```python
from build123d import *

# Parameters (mm, degrees)
SKETCH1_R                    = 4
SKETCH1_R_2                  = 1.5
EXTRUDE1_DEPTH               = 2
SKETCHED_START               = -63
SKETCHED_BEND1_OUTLINE_W     = 20
SKETCHED_BEND1_OUTLINE_H     = 2
SKETCHED_BEND1_DEPTH         = 35
SKETCHED_START_2             = -27.76405
SKETCHED_BEND1_2_OUTLINE_R   = 1.5
SKETCHED_BEND1_2_OUTLINE_R_2 = 4
SKETCHED_BEND1_2_DEPTH       = 1.76405
SKETCHED_START_3             = -28
SKETCHED_BEND1_3_OUTLINE_R   = 1.5
SKETCHED_BEND1_3_OUTLINE_R_2 = 4
SKETCHED_BEND1_3_DEPTH       = 2.5
SKETCHED_START_4             = -11
SKETCHED_BEND1_4_DEPTH       = 22


with BuildPart() as part:
    # Sketch1 → Extrude1 (new body)
    with BuildSketch(Plane.XY):
        with BuildLine():
            Line((0, -3), (0, -10))
            Line((0, -10), (-52, -10))
            ThreePointArc((-52, -10), (-62, 0), (-52, 10))
            Line((-52, 10), (0, 10))
            Line((0, 10), (0, 3))
            ThreePointArc((0, 3), (-3, 0), (0, -3))
        make_face()
        with Locations((-52, 0)):
            Circle(SKETCH1_R, mode=Mode.SUBTRACT)
        with Locations((-45, 0)):
            Circle(SKETCH1_R_2, mode=Mode.SUBTRACT)
        with Locations((-47.050252532, -4.949747468)):
            Circle(SKETCH1_R_2, mode=Mode.SUBTRACT)
        with Locations((-52, -7)):
            Circle(SKETCH1_R_2, mode=Mode.SUBTRACT)
        with Locations((-59, 0)):
            Circle(SKETCH1_R_2, mode=Mode.SUBTRACT)
        with Locations((-52, 7)):
            Circle(SKETCH1_R_2, mode=Mode.SUBTRACT)
        with Locations((-47.050252532, 4.949747468)):
            Circle(SKETCH1_R_2, mode=Mode.SUBTRACT)
        with Locations((-4.95, -4.95)):
            Circle(SKETCH1_R_2, mode=Mode.SUBTRACT)
        with Locations((-14.85, -4.95)):
            Circle(SKETCH1_R_2, mode=Mode.SUBTRACT)
        with Locations(Location((-4.95, 4.95, 0), (0, 0, 180))):
            Circle(SKETCH1_R_2, mode=Mode.SUBTRACT)
        with Locations(Location((-14.85, 4.95, 0), (0, 0, 180))):
            Circle(SKETCH1_R_2, mode=Mode.SUBTRACT)
    extrude(amount=EXTRUDE1_DEPTH)

    # Sketched Bend1: read off the stored shape, not the designer's step
    # Sketched Bend1 outline → Sketched Bend1 (cut)
    with BuildSketch(Plane.YZ.offset(SKETCHED_START)):
        with Locations((0, 1)):
            Rectangle(SKETCHED_BEND1_OUTLINE_W, SKETCHED_BEND1_OUTLINE_H)
    extrude(amount=SKETCHED_BEND1_DEPTH, mode=Mode.SUBTRACT)

    # Sketched Bend1 2 outline → Sketched Bend1 2 (add)
    with BuildSketch(Plane.YZ.offset(SKETCHED_START_2)):
        with BuildLine():
            Line((10, 2), (10, 26.64380551))
            ThreePointArc((10, 26.64380551), (0, 36.64380551), (-10, 26.64380551))
            Line((-10, 26.64380551), (-10, 2))
            Line((-10, 2), (10, 2))
        make_face()
        with Locations((-7, 26.64380551)):
            Circle(SKETCHED_BEND1_2_OUTLINE_R, mode=Mode.SUBTRACT)
        with Locations((-4.949747468, 21.694058042)):
            Circle(SKETCHED_BEND1_2_OUTLINE_R, mode=Mode.SUBTRACT)
        with Locations((0, 19.64380551)):
            Circle(SKETCHED_BEND1_2_OUTLINE_R, mode=Mode.SUBTRACT)
        with Locations((4.949747468, 21.694058042)):
            Circle(SKETCHED_BEND1_2_OUTLINE_R, mode=Mode.SUBTRACT)
        with Locations((0, 26.64380551)):
            Circle(SKETCHED_BEND1_2_OUTLINE_R_2, mode=Mode.SUBTRACT)
        with Locations((7, 26.64380551)):
            Circle(SKETCHED_BEND1_2_OUTLINE_R, mode=Mode.SUBTRACT)
        with Locations((0, 33.64380551)):
            Circle(SKETCHED_BEND1_2_OUTLINE_R, mode=Mode.SUBTRACT)
    extrude(amount=SKETCHED_BEND1_2_DEPTH)

    # Sketched Bend1 3 outline → Sketched Bend1 3 (add)
    with BuildSketch(Plane.YZ.offset(SKETCHED_START_3)):
        with BuildLine():
            Line((10, 2), (10, 26.64380551))
            ThreePointArc((10, 26.64380551), (0, 36.64380551), (-10, 26.64380551))
            Line((-10, 26.64380551), (-10, 2))
            Line((-10, 2), (10, 2))
        make_face()
        with Locations((-7, 26.64380551)):
            Circle(SKETCHED_BEND1_3_OUTLINE_R, mode=Mode.SUBTRACT)
        with Locations((-4.949747468, 21.694058042)):
            Circle(SKETCHED_BEND1_3_OUTLINE_R, mode=Mode.SUBTRACT)
        with Locations((0, 19.64380551)):
            Circle(SKETCHED_BEND1_3_OUTLINE_R, mode=Mode.SUBTRACT)
        with Locations((4.949747468, 21.694058042)):
            Circle(SKETCHED_BEND1_3_OUTLINE_R, mode=Mode.SUBTRACT)
        with Locations((0, 26.64380551)):
            Circle(SKETCHED_BEND1_3_OUTLINE_R_2, mode=Mode.SUBTRACT)
        with Locations((7, 26.64380551)):
            Circle(SKETCHED_BEND1_3_OUTLINE_R, mode=Mode.SUBTRACT)
        with Locations((0, 33.64380551)):
            Circle(SKETCHED_BEND1_3_OUTLINE_R, mode=Mode.SUBTRACT)
    extrude(amount=SKETCHED_BEND1_3_DEPTH)

    # Sketched Bend1 4 outline → Sketched Bend1 4 (cut)
    with BuildSketch(Plane(origin=(0, 0, 0), x_dir=(1, 0, 0), z_dir=(0, 1, 0)).offset(SKETCHED_START_4)):
        with BuildLine():
            Line((-26, -2.5), (-26, -38))
            Line((-26, -38), (-25.5, -38))
            Line((-25.5, -38), (-25.5, -2))
            ThreePointArc((-25.5, -2), (-25.853553391, -2.146446609), (-26, -2.5))
        make_face()
        with BuildLine():
            Line((-29, -38), (-27.999999998, -38))
            Line((-27.999999998, -38), (-28, -2.5))
            ThreePointArc((-28, -2.5), (-27.267766953, -0.732233047), (-25.5, 0))
            Line((-25.5, 0), (-24, 0))
            Line((-24, 0), (-24, 1))
            Line((-24, 1), (-29, 1))
            Line((-29, 1), (-29, -38))
        make_face()
    extrude(amount=SKETCHED_BEND1_4_DEPTH, mode=Mode.SUBTRACT)

    # Mirror1: part across plane


with BuildPart() as part_1:
    add(part.part)
    add(part.part.mirror(Plane(origin=(0, -3, 2), x_dir=(0, 0, 1), z_dir=(-1, 0, 0))))


solid = part_1.part
```
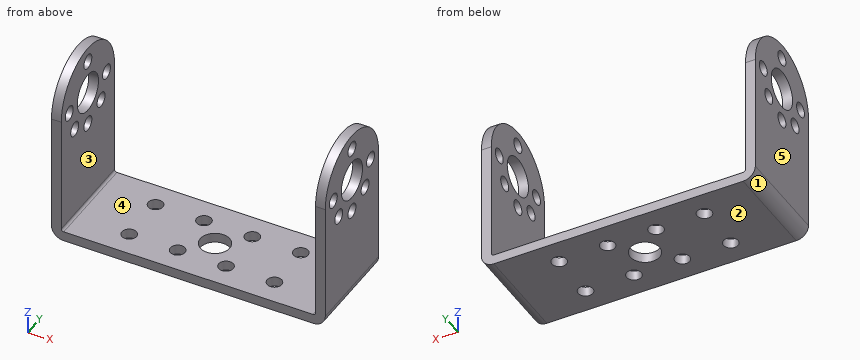
Work out the finished part from the listing and answer in its coordinate system (mm). Face numbers are marked on the shaded views. A direction names the side the tool comes from. Give positions to 0.01 mm unless a question says otherwise; leave off trailing zeros. Order: outer loops, then holes, each group sorted by start corner. A loop starts at its lowest first (then second) coordinate and runs counter-clockwise, first axis right, second up. Notation, with made-up numbers: (51, 59) - (107, 59) arc R25 ccw to (107, 82) - close; hole circle Ø8 at (53, 17). An arc over 180 degrees is marked (long way). One line per item, written item: value. Start each with the question number.
1. Section D-D, the plane y = 0 is taken. Count the separate pieces of the cut face and the enclosed holes in it, then the cut area to 3 significant figures.
2. Section C-C, the plane y = 7.75 is taken. Write down the section's boundary in (x, z), then the cut area to 3 significant figures.
3. Section B-B, the plane z = 11 is taken. Write down the section's boundary in (x, y), then the cut area to 3 significant figures.
4. Section A-A, the plane x = 14.85 is taken. Write down the section's boundary in (y, z), then the cut area to 3 significant figures.
5. This flat-tipped pin is pushed along its axis until it touches: pin 1 Ø6 at (x, y) = (5, -4) entering from +Z. Where does it stop, or does it pass through?
6. Consider line 1 (Y direction, x = -4.95, z = 1.65); line 2 (X direction, y = -1, z = 3.5); line 3 (X direction, y = 4.95, z = 0.7). Determine where each line is inside the solid, lowest interval first.
7. For a pull along X with two mould halves and no side action, classify the marked faces 1, 2 and 3 as released by +X, released by -X, zero draft, split by the parting line, or undercut.
8. Which of the six approach directions +Z, -Z, +X, -X, +Y, -Y give full straight-line access (tool end or side, diameter ignored) to the marked faces 4 and 5?
Filled sheet:
1. separate pieces: 8
1. enclosed holes: 0
1. area: 180 mm²
2. outline: (-28, 2.5) arc R2.5 ccw to (-25.5, 0) - (25.5, 0) arc R2.5 ccw to (28, 2.5) - (28, 25.34) - (26, 25.34) - (26, 2.5) arc R0.5 cw to (25.5, 2) - (-25.5, 2) arc R0.5 cw to (-26, 2.5) - (-26, 25.34) - (-28, 25.34) - close; (-28, 27.94) - (-26, 27.94) - (-26, 32.96) - (-28, 32.96) - close; (26, 27.94) - (28, 27.94) - (28, 32.96) - (26, 32.96) - close
2. area: 223 mm²
3. outline: (-28, -10) - (-26, -10) - (-26, 10) - (-28, 10) - close; (26, -10) - (28, -10) - (28, 10) - (26, 10) - close
3. area: 80.0 mm²
4. outline: (-10, 0) - (-6.45, 0) - (-6.45, 2) - (-10, 2) - close; (-3.45, 0) - (3.45, 0) - (3.45, 2) - (-3.45, 2) - close; (6.45, 0) - (10, 0) - (10, 2) - (6.45, 2) - close
4. area: 28.0 mm²
5. pin 1: z = 2
6. line 1: -10 to -6.45, -3.45 to 3.45, 6.45 to 10
6. line 2: -28 to -26, 26 to 28
6. line 3: -27.23 to -16.35, -13.35 to -6.45, -3.45 to 3.45, 6.45 to 13.35, 16.35 to 27.23
7. face 1: released by -X
7. face 2: zero draft
7. face 3: undercut
8. face 4: +Z, +Y, -Y
8. face 5: +Z, -Z, -X, +Y, -Y
